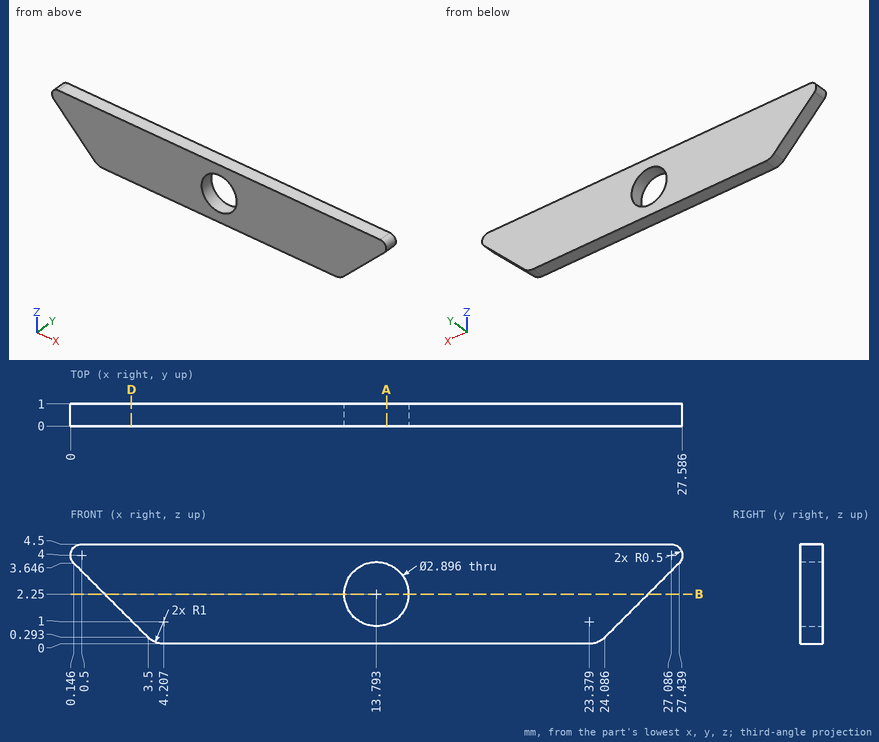
Source: three-view drawing plus pictorial views. Frame: mm from the lowest corner of the part. Round coordinates to 2 decimals unless told otherwise and drop trailing zeros. Write each loop counter-clockwise with the first axis right and the second up, starting at its lowest first coordinate (ties: lowest second). Pieces come first, ordered by that corner, then holes. Notation, with made-up numbers: (74.5, 53) -> (83.5, 53) arc R22 cw to (83.5, 80) -> close; hole circle Ø3 at (47.5, 89.25). An arc over 180 degrees is marked (long way). Return JSON: item names as keys, results as strings.
Q1. Section A-A on x = 14.25. Return the cut outline in (y, z).
From the geometry:
{"outline": "(0, 0) -> (1, 0) -> (1, 0.88) -> (0, 0.88) -> close; (0, 3.62) -> (1, 3.62) -> (1, 4.5) -> (0, 4.5) -> close"}
Q2. Section D-D on x = 2.75. Return the cut outline in (y, z).
From the geometry:
{"outline": "(0, 1.04) -> (1, 1.04) -> (1, 4.5) -> (0, 4.5) -> close"}
Q3. Section B-B on z = 2.25. Return the cut outline in (x, y) (1 decimal).
From the geometry:
{"outline": "(1.5, 0) -> (12.3, 0) -> (12.3, 1) -> (1.5, 1) -> close; (15.2, 0) -> (26, 0) -> (26, 1) -> (15.2, 1) -> close"}
Q4. Ray query, line 1 (X direction, y = 0.35, z = 2.25) (1 decimal); line 2 (Z direction, x = 13, y = 0.4); line 3 (Z direction, x = 14, y = 0.8). Return the intervals inside material, ascending.
From the geometry:
{"line 1": "1.5 to 12.3, 15.2 to 26", "line 2": "0 to 1.04, 3.46 to 4.5", "line 3": "0 to 0.82, 3.68 to 4.5"}
